Check sheet for the modelled part. Datum: model origin and axes. Units: mm. Face numbers are marked on the shaded views. A direction names the side the tool comes from. Give positions to 0.01 mm unless a question says otherwise; leave off trailing zeros. Loops run counter-clockwise (first coordinate to the right, second up) from the corner with the lowest first, then second, coordinate; pieces in that order, holes last. Notation, with made-up numbers: (-16.75, 64) -> (-11.75, 64) arc R19 cw to (-11.75, 86) -> close; hole circle Ø8 at (34, 58). An arc over 180 degrees is marked (long way). Write each question's results on one line, items separated by ' | '. Start each with the question number.
1. Tool access check on the marked faces 1 and 2. Record the directions out of +Z, -Z, +X, -X, +Y, -Y that give a thin tool (end or side, any length) a straight path to the whole face; none if there is none.
2. Material ranges on L1, parallel to Z at x = 5, y = -14.5; L2, parallel to Y at x = -8.5, z = -4; L3, parallel to Y at x = 2.5, z = -12, recorded low to high. Write a range as from..to.
3. Cross-section at A-A on x = 0. Record the boundary of the cut face in (y, z), and give its area (3 significant figures).
4. Cross-section at B-B on z = -15.5. Record the boundary of the cut face in (x, y), and give its area (3 significant figures).
5. Gauge pin test, flat ends, axial feed: pin 1 Ø4 at (x, y) = (-14, 6.5) entering from -Z; pin 2 Ø6 at (y, z) = (1.5, -7) entering from +X; pin 3 Ø10 at (y, z) = (4.5, -11) entering from -X. Record the tip position at first contact, or that the pin passes through.
6. Cross-section at C-C on y = -16. Record the boundary of the cut face in (x, z), and give its area (3 significant figures).
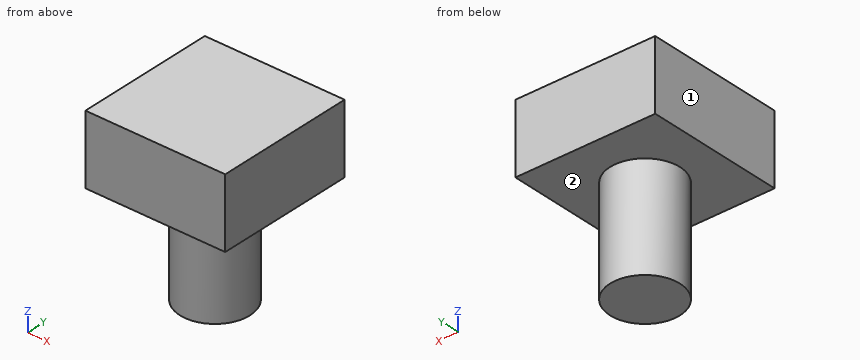
from build123d import *

# Parameters (mm, degrees)
F0_W     = 40
F0_H     = 40
F1_DEPTH = 20
F2_R     = 10
F3_DEPTH = 50


with BuildPart() as f1:
    # F0 (on Top) → F1 (new body)
    with BuildSketch(Plane.XY):
        Rectangle(F0_W, F0_H)
    extrude(amount=F1_DEPTH)

    # F2 (on face) → F3 (join)
    with BuildSketch(Plane.XY.offset(20)):
        Circle(F2_R)
    extrude(amount=-F3_DEPTH)


solid = f1.part
Geometry says:
1) face 1: +Z, -Z, -X, +Y, -Y | face 2: -Z
2) L1: 0..20 | L2: -5.27..5.27 | L3: -9.68..9.68
3) outline: (-20, 0) -> (-10, 0) -> (-10, -30) -> (10, -30) -> (10, 0) -> (20, 0) -> (20, 20) -> (-20, 20) -> close | area: 1,400 mm^2
4) outline: circle Ø20 at (0, 0) | area: 314 mm^2
5) pin 1: z = 0 | pin 2: x = 10 | pin 3: x = -10
6) outline: (-20, 0) -> (20, 0) -> (20, 20) -> (-20, 20) -> close | area: 800 mm^2
